Read the model definition and answer for the solid it produces. Units are mm, in the model's axes. Round coordinates to 2 decimals unless told otherwise and drop trailing zeros. Order: outer loops, then holes, each group sorted by start corner. A loop starts at its lowest first (then second) coordinate and runs counter-clockwise, first axis right, second up. Notation, with made-up numbers: (-40, 18) - (-10, 18) arc R22 ccw to (-10, 37) - close; hole circle Ø2 at (-40, 42.5). An arc over 180 degrees is marked (long way). One line per question, with ' | ' between items. Start each with the question number.
1) The part is cut by section D-D, the plane z = 10.25. Count the separate pieces of the cut face and the enclosed holes in it, plus the area to 3 significant figures.
2) Straight lines are drawn through the part: line 1 (X direction, y = 88, z = 12.25); line 2 (X direction, y = -23, z = 6.25); line 3 (X direction, y = -9, z = 13.25). For each, find the intervals that lie inside material, in ascending order. Write a range as from..to.
3) Flat-ended cylindrical pins translate along their axes: pin 1 (5 mm diameter, centred on x = 140, z = 10, fed in from -Y); pin 2 (4 mm diameter, centred on y = -24, z = 9.5, fed in from +X); pin 3 (10 mm diameter, centred on x = -48.5, z = 9.5, fed in from +Y). Find the tip coordinate at first contact, or state that the pin passes through.
4) The part is cut by section B-B, the plane x = -112.5. Give the vertices of the cut face in (y, z), plus the area to 3 significant figures.
5) The part is cut by section C-C, the plane x = 49.5. Give the vertices of the cut face in (y, z), plus the area to 3 significant figures.
6) The part is cut by section A-A, the plane y = 145. Give the vertices of the cut face in (x, z).
from build123d import *

# Parameters (mm, degrees)
SKETCH1_W           = 17
SKETCH1_H           = 30
BOSS_EXTRUDE1_DEPTH = 17


with BuildPart() as part:
    # Sketch1 → Boss-Extrude1 (new body)
    with BuildSketch(Plane.XY):
        with BuildLine():
            Line((-125, -170), (-87, -170))
            Line((-87, -170), (-87, -140))
            Line((-87, -140), (-70, -140))
            Line((-70, -140), (-70, -170))
            Line((-70, -170), (-40, -170))
            Line((-40, -170), (40, -170))
            Line((40, -170), (70, -170))
            Line((70, -170), (70, -140))
            Line((70, -140), (87, -140))
            Line((87, -140), (87, -170))
            Line((87, -170), (125, -170))
            ThreePointArc((125, -170), (139.142135624, -164.142135624), (145, -150))
            Line((145, -150), (145, -50))
            Line((145, -50), (125, -50))
            ThreePointArc((125, -50), (110.857864376, -44.142135624), (105, -30))
            Line((105, -30), (105, 0))
            Line((105, 0), (105, 30))
            ThreePointArc((105, 30), (110.857864376, 44.142135624), (125, 50))
            Line((125, 50), (145, 50))
            Line((145, 50), (145, 150))
            ThreePointArc((145, 150), (139.142135624, 164.142135624), (125, 170))
            Line((125, 170), (87, 170))
            Line((87, 170), (87, 140))
            Line((87, 140), (70, 140))
            Line((70, 140), (70, 170))
            Line((70, 170), (40, 170))
            Line((40, 170), (40, 181.8))
            Line((40, 181.8), (10, 181.8))
            Line((10, 181.8), (10, 170))
            Line((10, 170), (-10, 170))
            Line((-10, 170), (-10, 181.8))
            Line((-10, 181.8), (-40, 181.8))
            Line((-40, 181.8), (-40, 170))
            Line((-40, 170), (-70, 170))
            Line((-70, 170), (-70, 140))
            Line((-70, 140), (-87, 140))
            Line((-87, 140), (-87, 170))
            Line((-87, 170), (-125, 170))
            ThreePointArc((-125, 170), (-139.142135624, 164.142135624), (-145, 150))
            Line((-145, 150), (-145, 50))
            Line((-145, 50), (-125, 50))
            ThreePointArc((-125, 50), (-110.857864376, 44.142135624), (-105, 30))
            Line((-105, 30), (-105, 0))
            Line((-105, 0), (-105, -30))
            ThreePointArc((-105, -30), (-110.857864376, -44.142135624), (-125, -50))
            Line((-125, -50), (-145, -50))
            Line((-145, -50), (-145, -150))
            ThreePointArc((-145, -150), (-139.142135624, -164.142135624), (-125, -170))
        make_face()
        with Locations((-78.5, -95)):
            Rectangle(SKETCH1_W, SKETCH1_H, mode=Mode.SUBTRACT)
        with Locations((-78.5, -35)):
            Rectangle(SKETCH1_W, SKETCH1_H, mode=Mode.SUBTRACT)
        with Locations((-78.5, 35)):
            Rectangle(SKETCH1_W, SKETCH1_H, mode=Mode.SUBTRACT)
        with Locations((78.5, 95)):
            Rectangle(SKETCH1_W, SKETCH1_H, mode=Mode.SUBTRACT)
        with Locations((-78.5, 95)):
            Rectangle(SKETCH1_W, SKETCH1_H, mode=Mode.SUBTRACT)
        with Locations((78.5, 35)):
            Rectangle(SKETCH1_W, SKETCH1_H, mode=Mode.SUBTRACT)
        with Locations((78.5, -35)):
            Rectangle(SKETCH1_W, SKETCH1_H, mode=Mode.SUBTRACT)
        with Locations((78.5, -95)):
            Rectangle(SKETCH1_W, SKETCH1_H, mode=Mode.SUBTRACT)
    extrude(amount=BOSS_EXTRUDE1_DEPTH)


solid = part.part
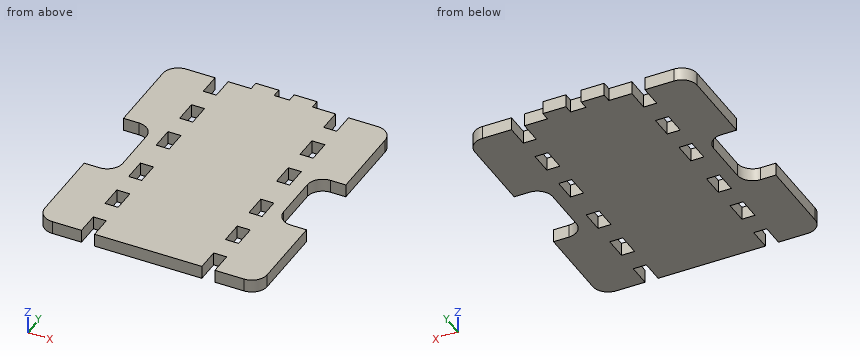
Values:
1) separate pieces: 1 | enclosed holes: 8 | area: 85,200 mm^2
2) line 1: x = -145..-87, -70..70, 87..145 | line 2: x = -105..-87, -70..70, 87..105 | line 3: x = -105..105
3) pin 1: stops at y = -165.61 | pin 2: stops at x = 105 | pin 3: stops at y = 170
4) outline: (-170, 0) - (-45.61, 0) - (-45.61, 17) - (-170, 17) - close; (45.61, 0) - (170, 0) - (170, 17) - (45.61, 17) - close | area: 4,230 mm^2
5) outline: (-170, 0) - (170, 0) - (170, 17) - (-170, 17) - close | area: 5,780 mm^2
6) outline: (-145, 0) - (-87, 0) - (-87, 17) - (-145, 17) - close; (-70, 0) - (70, 0) - (70, 17) - (-70, 17) - close; (87, 0) - (145, 0) - (145, 17) - (87, 17) - close
